```python
from build123d import *

# Parameters (mm, degrees)
ESTRUSIONE_ESTRUSIONE1_DEPTH                         = 15
TAGLIO_ESTRUSIONE1_DEPTH                             = 3
FORO_LAMATO_PER_VITE_M6_A_TESTA_CILINDRI_D           = 6.4
FORO_LAMATO_PER_VITE_M6_A_TESTA_CILINDRI_CBORE_D     = 11
FORO_LAMATO_PER_VITE_M6_A_TESTA_CILINDRI_CBORE_DEPTH = 6.4
RIPETIZIONECIRCOLARE1_COUNT                          = 2
FORO_PER_VITE_M6_1_D                                 = 6.6


with BuildPart() as part:
    # Schizzo1 → Estrusione-Estrusione1 (new body)
    with BuildSketch(Plane(origin=(0, -3, 0), x_dir=(1, 0, 0), z_dir=(0, 1, 0))):
        with BuildLine():
            Line((198.9, -65), (-132.5, -65))
            ThreePointArc((-132.5, -65), (-139.571067812, -62.071067812), (-142.5, -55))
            Line((-142.5, -55), (-142.5, 55))
            ThreePointArc((-142.5, 55), (-139.571067812, 62.071067812), (-132.5, 65))
            Line((-132.5, 65), (198.9, 65))
            ThreePointArc((198.9, 65), (205.971067812, 62.071067812), (208.9, 55))
            Line((208.9, 55), (208.9, -55))
            ThreePointArc((208.9, -55), (205.971067812, -62.071067812), (198.9, -65))
        make_face()
    extrude(amount=ESTRUSIONE_ESTRUSIONE1_DEPTH)

    # Schizzo2 → Taglio-Estrusione1 (cut)
    with BuildSketch(Plane(origin=(0, -3, 0), x_dir=(1, 0, 0), z_dir=(0, 1, 0))):
        with BuildLine():
            Line((149.372135955, 42.749691048), (208.9, 42.749691048))
            Line((208.9, 42.749691048), (208.9, -42.749691048))
            Line((208.9, -42.749691048), (149.372135955, -42.749691048))
            ThreePointArc((149.372135955, -42.749691048), (148.555639374, -42.92394919), (147.88142397, -43.416357715))
            ThreePointArc((147.88142397, -43.416357715), (142.071572875, -43.578118173), (142.233333333, -37.768267078))
            ThreePointArc((142.233333333, -37.768267078), (142.725741858, -37.094051674), (142.9, -36.277555093))
            Line((142.9, -36.277555093), (142.9, 36.277555093))
            ThreePointArc((142.9, 36.277555093), (142.725741858, 37.094051674), (142.233333333, 37.768267078))
            ThreePointArc((142.233333333, 37.768267078), (142.071572875, 43.578118173), (147.88142397, 43.416357715))
            ThreePointArc((147.88142397, 43.416357715), (148.555639374, 42.92394919), (149.372135955, 42.749691048))
        make_face()
    taglio_estrusione1 = extrude(amount=TAGLIO_ESTRUSIONE1_DEPTH, mode=Mode.SUBTRACT)

    # Foro lamato per Vite M6 a testa cilindri (through all)
    with Locations(Plane(origin=(0, 12, 0), x_dir=(1, 0, 0), z_dir=(0, 1, 0))):
        with Locations((154.9, -28.899213583), (154.9, 14.100786417), (196.9, 14.100786417)):
            foro_lamato_per_vite_m6_a_testa_cilindri = CounterBoreHole(FORO_LAMATO_PER_VITE_M6_A_TESTA_CILINDRI_D / 2, FORO_LAMATO_PER_VITE_M6_A_TESTA_CILINDRI_CBORE_D / 2, FORO_LAMATO_PER_VITE_M6_A_TESTA_CILINDRI_CBORE_DEPTH)

    # Specchia1: Taglio-Estrusione1 across plane
    add(taglio_estrusione1.mirror(Plane(origin=(33.2, 0, 0), x_dir=(0, 0, 1), z_dir=(1, 0, 0))), mode=Mode.SUBTRACT)

    # RipetizioneCircolare1: Foro lamato per Vite M6 a testa cilindri ×2 about axis
    ripetizionecircolare1_axis = Axis((33.2, 0, 0), (0, 1, 0))
    for i in range(1, RIPETIZIONECIRCOLARE1_COUNT):
        add(foro_lamato_per_vite_m6_a_testa_cilindri.rotate(ripetizionecircolare1_axis, i * 360 / RIPETIZIONECIRCOLARE1_COUNT), mode=Mode.SUBTRACT)

    # Foro per Vite M6-1 (through all)
    with Locations(Plane(origin=(0, -3, 0), x_dir=(-1, 0, 0), z_dir=(0, -1, 0))):
        with Locations((-133.2, 25), (66.8, -25), (66.8, 25), (-133.2, -25), (-33.2, -25), (-33.2, 25), (16.8, -25), (16.8, 25), (-83.2, 25), (-83.2, -25)):
            Hole(FORO_PER_VITE_M6_1_D / 2)


solid = part.part
```
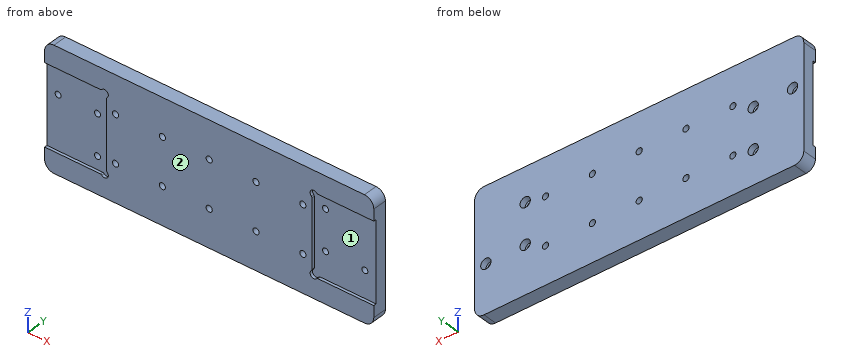
Could you check a few things on this model? Use its own coordinates, in mm. Face numbers are marked on the shaded views. Give positions to 0.01 mm unless a question says otherwise; leave off trailing zeros. Loops run counter-clockwise (first coordinate to the right, second up) from the corner with the lowest first, then second, coordinate; pieces in that order, holes last. Notation, with made-up numbers: (19, 28) - (76, 28) arc R20 ccw to (76, 50) - close; hole circle Ø2 at (89, -22.75). An arc over 180 degrees is marked (long way). Use one line per item in the form item = value.
1. I want a section at B-B (z = -5). Please give me the cut outline in (x, y), and give its area (4 significant figures).
Response values:
outline = (-142.5, 0) - (-76.5, 0) - (-76.5, -3) - (142.9, -3) - (142.9, 0) - (208.9, 0) - (208.9, 12) - (-142.5, 12) - close
area = 4,875 mm²
2. Thinking about a two-plate mould opening in Z: for the marked faces 1 and 2, which applies, released by +Z, released by -Z, zero draft, split by the parting line, or undercut?
Response values:
face_1 = undercut
face_2 = zero draft
3. I want a section at C-C (x = 133.2). Please give me the cut outline in (y, z).
Response values:
outline = (-3, -65) - (12, -65) - (12, -28.3) - (-3, -28.3) - close; (-3, -21.7) - (12, -21.7) - (12, 21.7) - (-3, 21.7) - close; (-3, 28.3) - (12, 28.3) - (12, 65) - (-3, 65) - close
4. I'm going to push flat-ended pins straight in: pin 1 Ø6 at (x, z) = (-130.5, 14.1) entering from +Y; pin 2 Ø12 at (x, z) = (156, 31) entering from +Y; pin 3 Ø17.5 at (x, z) = (196.9, -14.1) entering from -Y; pin 4 Ø8.5 at (x, z) = (-88.5, -28.9) entering from +Y. Where does each tip first touch, or does it pass through?
Response values:
pin_1 = through
pin_2 = 12
pin_3 = 0
pin_4 = 5.6
5. I need wall thicknesses on probe 1 along X at (y, z) = (3, 25); probe 2 along X at (y, z) = (4.25, 22); probe 3 along X at (y, z) = (-2, 43.5). Which ranges of each line are inside material? Lowest first, please.
Response values:
probe_1 = -142.5 to -70.1, -63.5 to -20.1, -13.5 to 29.9, 36.5 to 79.9, 86.5 to 129.9, 136.5 to 208.9
probe_2 = -142.5 to -68.17, -65.43 to -18.17, -15.43 to 31.83, 34.57 to 81.83, 84.57 to 131.83, 134.57 to 208.9
probe_3 = -142.5 to -81.4, -75.6 to 142, 147.8 to 208.9
6. I want a section at A-A (x = -88.5). Please give me the cut outline in (y, z), and give its area (3 significant figures).
Response values:
outline = (-3, -65) - (12, -65) - (12, -34.4) - (5.6, -34.4) - (5.6, -32.1) - (0, -32.1) - (0, -42.75) - (-3, -42.75) - close; (-3, 42.75) - (0, 42.75) - (0, 17.3) - (5.6, 17.3) - (5.6, 19.6) - (12, 19.6) - (12, 65) - (-3, 65) - close; (0, -25.7) - (5.6, -25.7) - (5.6, -23.4) - (12, -23.4) - (12, 8.6) - (5.6, 8.6) - (5.6, 10.9) - (0, 10.9) - close
area = 1,480 mm²
